```python
from build123d import *

# Parameters (mm, degrees)
SKETCH1_R           = 45
SKETCH1_R_2         = 30
BOSS_EXTRUDE1_DEPTH = 3
CUT_EXTRUDE1_DEPTH  = 1.5
CIRPATTERN1_COUNT   = 5


with BuildPart() as part:
    # Sketch1 → Boss-Extrude1 (new body)
    with BuildSketch(Plane(origin=(0, 0, 0), x_dir=(1, 0, 0), z_dir=(0, 1, 0))):
        Circle(SKETCH1_R)
        Circle(SKETCH1_R_2, mode=Mode.SUBTRACT)
    extrude(amount=BOSS_EXTRUDE1_DEPTH)

    # Sketch2 → Cut-Extrude1 (cut)
    with BuildSketch(Plane(origin=(0, 3, 0), x_dir=(1, 0, 0), z_dir=(0, 1, 0))):
        with BuildLine():
            Line((10, 34.438191534), (-22.713965574, 34.438191534))
            ThreePointArc((-22.713965574, 34.438191534), (-23.338965574, 35.063191534), (-22.713965574, 35.688191534))
            Line((-22.713965574, 35.688191534), (10, 35.688191534))
            ThreePointArc((10, 35.688191534), (10.625, 35.063191534), (10, 34.438191534))
        make_face()
    cut_extrude1 = extrude(amount=-CUT_EXTRUDE1_DEPTH, mode=Mode.SUBTRACT)

    # CirPattern1: Cut-Extrude1 ×5 about axis
    cirpattern1_axis = Axis((0, 0, 0), (0, 1, 0))
    for i in range(1, CIRPATTERN1_COUNT):
        add(cut_extrude1.rotate(cirpattern1_axis, i * 360 / CIRPATTERN1_COUNT), mode=Mode.SUBTRACT)


solid = part.part
```
Geometry check sheet. Reference: the model listing, model coordinates, mm. A direction names the side the tool comes from. Round coordinates to 2 decimals unless told otherwise and drop trailing zeros. Order: outer loops, then holes, each group sorted by start corner. A loop starts at its lowest first (then second) coordinate and runs counter-clockwise, first axis right, second up. Notation, with made-up numbers: M 33.25,-39 L 61.25,-39 A24 ccw 61.25,-4 Z; hole C -23,-4.75 d7. An arc over 180 degrees is marked long. Write item = value, one per line.
Q1. Section check C-C (z = 36.5). Enter the section's corners in (x, y).
Answer block:
outline = M -26.32,0 L 26.32,0 L 26.32,3 L -8.35,3 L -8.35,1.5 L -10.48,1.5 L -10.48,3 L -26.32,3 Z
Q2. Scan lines: line 1 (Z direction, x = 0, y = 2.4); line 2 (Z direction, x = -24, y = 1.9); line 3 (X direction, y = 2.35, z = 0). Record each from-to range of solid material in increasing order.
Answer block:
line_1 = -45 to -35.69, -34.44 to -30, 30 to 45
line_2 = -38.07 to -18, 18 to 25.13, 26.68 to 38.07
line_3 = -45 to -37.52, -36.21 to -30, 30 to 45
Q3. Set-up check for faces 4 (the flat face through (31, 1.5, -17)), 5 (the flat face through (29, 0, 9)): record each of +Z, -Z, +X, -X, +Y, -Y from which the full face is reachable in a straight line by a thin tool's end or side.
Answer block:
face_4 = +Y
face_5 = +Z, -Z, +X, -X, -Y
Q4. Depth check by flat-ended pin: pin 1 Ø1.2 at (x, y) = (-11, 2.5) entering from -Z; pin 2 Ø1 at (x, z) = (-0.5, -35) entering from +Y; pin 3 Ø1.2 at (x, y) = (-13.5, 2.5) entering from +Z. Enter the tip coordinate at first touch or a pass-through.
Answer block:
pin_1 = -43.78
pin_2 = 1.5
pin_3 = 43.11
Q5. Section check D-D (x = -37.5). Enter the section's corners in (y, z).
Answer block:
outline = M 0,-24.87 L 3,-24.87 L 3,-0.08 L 1.5,-0.08 L 1.5,3.97 L 3,3.97 L 3,24.87 L 0,24.87 Z
Q6. Section check A-A (x = 0). Enter the section's corners in (y, z), plus the area to 3 significant figures.
Answer block:
outline = M 0,-45 L 3,-45 L 3,-35.69 L 1.5,-35.69 L 1.5,-34.44 L 3,-34.44 L 3,-30 L 0,-30 Z; M 0,30 L 3,30 L 3,45 L 0,45 Z
area = 88.1 mm^2
Q7. Section check B-B (y = 2.45). Give the number of separate pieces and of enclosed holes in the cut face, plus the area to 3 significant figures.
Answer block:
separate_pieces = 1
enclosed_holes = 6
area = 3,320 mm^2
Q8. Release check for a two-part mould opening along X. For faces 1 (the flat face through (26.31, 2.26, 25)), 2 (the flat face through (29, 3, 9)), 3 (the cylindrical face through (20.765, 1.479, 39.923)) record: released by +X, released by -X, zero draft, split by the parting line, or undercut.
Answer block:
face_1 = undercut
face_2 = zero draft
face_3 = split by the parting line
